Study the drawing (mm; zero at the part's minimum x, y, z) and answer. A direction names the side the tool comes from. Give positions to 0.01 mm unless a question says otherwise; leave off trailing zeros. Use a Markdown table: item, result. Add a question column.
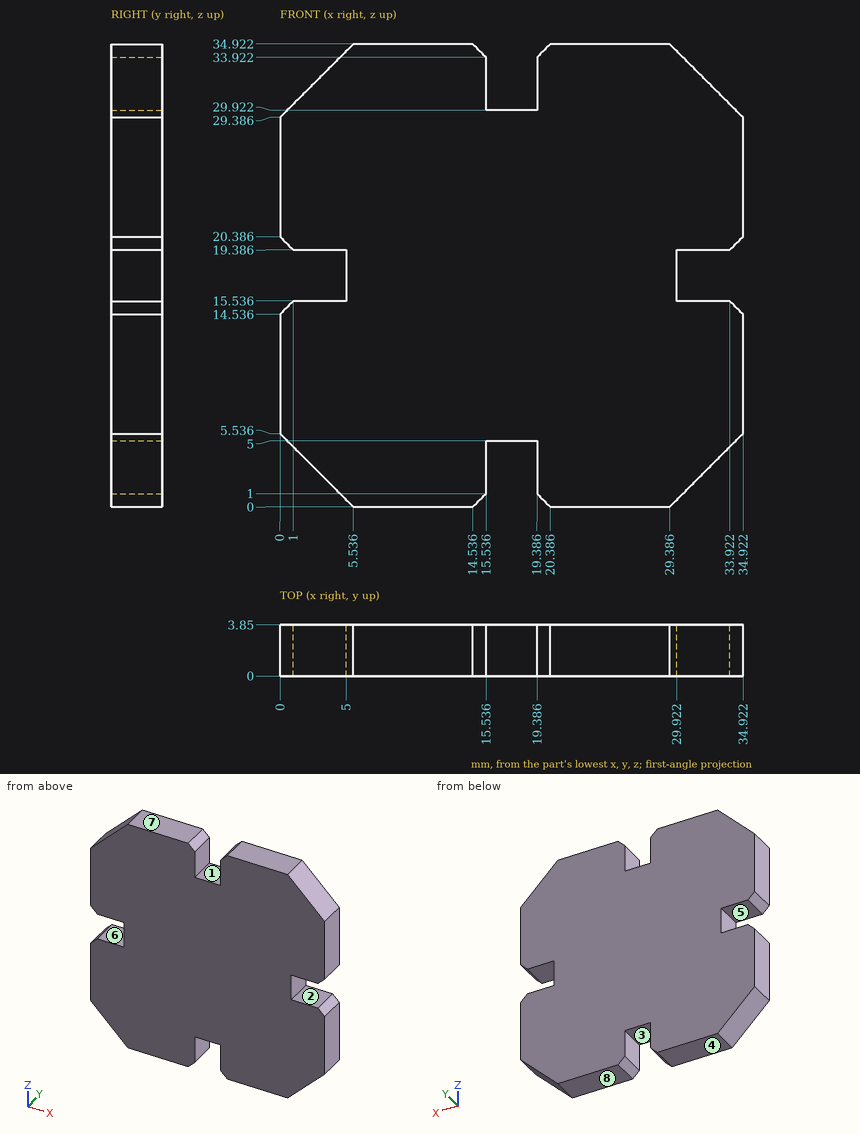
1) Straight lines are drawn through the part: line 1 (Z direction, x = 16.5, y = 2.25); line 2 (Z direction, x = 4, y = 3.5) (1 decimal); line 3 (X direction, y = 3.5, z = 31) (1 decimal). For each, find the intervals that lie inside material, in ascending order.
2) Which of the six approach directions +Z, -Z, +X, -X, +Y, -Y give full straight-line access (tool end or side, diameter ignored) to the marked faces 1, 2, 3, 4 and 5?
3) Determine the mould class of the marked faces 6, 7 and 8 for opening direction Z: released by +Z, released by -Z, zero draft, split by the parting line, or undercut.
4) Flat-ended cylindrical pins translate along their axes: pin 1 (1.2 mm diameter, centred on y = 1.5, z = 3, fed in from +X) (1 decimal); pin 2 (1.9 mm diameter, centred on x = 17, y = 2.5, fed in from -Z); pin 3 (1.9 mm diameter, centred on x = 18.5, y = 2.5, fed in from +Z) (1 decimal). Find the tip coordinate at first contact, or state that the pin passes through.
A:
| question | item | result |
|---|---|---|
| 1 | line 1 | 5 to 29.92 |
| 1 | line 2 | 1.5 to 15.5, 19.4 to 33.4 |
| 1 | line 3 | 1.6 to 15.5, 19.4 to 33.3 |
| 2 | face 1 | +Z, +Y, -Y |
| 2 | face 2 | +X, +Y, -Y |
| 2 | face 3 | -Z, +Y, -Y |
| 2 | face 4 | -Z, +X, -X, +Y, -Y |
| 2 | face 5 | -X, +Y, -Y |
| 3 | face 6 | undercut |
| 3 | face 7 | released by +Z |
| 3 | face 8 | released by -Z |
| 4 | pin 1 | x = 33 |
| 4 | pin 2 | z = 5 |
| 4 | pin 3 | z = 34 |
